Autodesk Inventor part; units mm, degrees
ref_plane "YZ Plane" through (0, 0, 0) normal (1, 0, 0) x (0, 1, 0)
ref_plane "XZ Plane" through (0, 0, 0) normal (0, 1, 0) x (-1, 0, 0)
ref_plane "XY Plane" through (0, 0, 0) normal (0, 0, 1) x (1, 0, 0)
ref_plane "Work Plane1" through (44.003, -30.6729, -33.7942) normal (0, 0, 1) x (1, 0, 0)
sketch "Sketch1" plane through (44.003, -30.6729, -33.7942) normal (0, 0, 1) x (1, 0, 0)
  line L0 (145, 55) -> (160, 55)
  arc A0 (145, 55) -> (135, 45) centre (145, 45) ccw
  line L1 (135, 30) -> (135, 45)
  arc A1 (135, 30) -> (145, 20) centre (145, 30) ccw
  line L2 (160, 20) -> (145, 20)
  arc A2 (160, 20) -> (170, 30) centre (160, 30) ccw
  line L3 (170, 45) -> (170, 30)
  arc A3 (170, 45) -> (160, 55) centre (160, 45) ccw
  point P0 (-44.003, 30.6729)
surface extrude "ExtrusionSrf1" sketch "Sketch1" along normal blind 20 shown yes curves A3 L0 A0 L1 A1 L2 A2 L3
thicken "Thicken1" operation new thickness 3 both sides no extend neighbours no toward (-0.7330519, 0.6801727, 0) faces at (211.3335, -7.4746, -20.4609) (214.003, 4.3271, -27.1276) (210.8047, 21.6576, -20.4609) (199.003, 24.3271, -27.1276) (181.6724, 21.1289, -20.4609) (179.003, 9.3271, -27.1276) (188.2557, -10.6449, -20.4609) (194.003, -10.6729, -27.1276)
properties part number "CE-8.2.2-01-004"
CAD build for the part. Positions are in the model's coordinates, mm. A direction names the side the tool comes from. Coordinates: 2 decimals unless noted, no trailing zeros. Order: outer loops, then holes, each group sorted by start corner. A loop starts at its lowest first (then second) coordinate and runs counter-clockwise, first axis right, second up.
(1) Drill centre lines: L1, parallel to Y at x = 199, z = -21; L2, parallel to X at y = 6.5, z = -15.25; L3, parallel to X at y = -4, z = -24.25. Where is each one in solid material? Low to high.
Solution:
L1: y = -10.67 to -7.67, 21.33 to 24.33
L2: x = 179 to 182, 211 to 214
L3: x = 179.57 to 182.84, 210.16 to 213.43
(2) Saw through at A-A, the plane x = 200. Write the cut outline in (y, z), and give its area (3 significant figures).
Solution:
outline: (-10.67, -33.79) - (-7.67, -33.79) - (-7.67, -13.79) - (-10.67, -13.79) - close; (21.33, -33.79) - (24.33, -33.79) - (24.33, -13.79) - (21.33, -13.79) - close
area: 120 mm2
(3) Mould opens along X. For faces 1 (the face through (214.003, 7, -24)), 2 (the face through (179.003, 7, -24)), 3 (the face through (209.007, -5.568, -23.934)) say: released by +X, released by -X, zero draft, split by the parting line, or undercut.
Solution:
face 1: released by +X
face 2: released by -X
face 3: undercut
(4) Saw through at C-C, the plane z = -25.5. Write the cut outline in (x, y), and give its area (3 significant figures).
Solution:
outline: (179, -0.67) arc R10 ccw to (189, -10.67) - (204, -10.67) arc R10 ccw to (214, -0.67) - (214, 14.33) arc R10 ccw to (204, 24.33) - (189, 24.33) arc R10 ccw to (179, 14.33) - close; hole (182, -0.67) arc R7 ccw to (189, -7.67) - (204, -7.67) arc R7 ccw to (211, -0.67) - (211, 14.33) arc R7 ccw to (204, 21.33) - (189, 21.33) arc R7 ccw to (182, 14.33) - close
area: 340 mm2
(5) Which spindle directions (+Z, -Z, +X, -X, +Y, -Y) get a long thin tool onto all of the face, cutting with end or side? Do faces 4 (the face through (182.01, -7.82, -23.93)), 5 (the face through (183.999, 19.222, -23.934)). Say none if no direction does.
Solution:
face 4: +Z, -Z, -X, -Y
face 5: +Z, -Z
(6) Saw through at B-B, the plane y = 11. Write the cut outline in (x, z).
Solution:
outline: (179, -33.79) - (182, -33.79) - (182, -13.79) - (179, -13.79) - close; (211, -33.79) - (214, -33.79) - (214, -13.79) - (211, -13.79) - close
(7) Pin check, flat tip, straight feed: pin 1 Ø3 at (y, z) = (17, -26.5) entering from -X. Stop position of the tip, or through.
Solution:
pin 1: stops at x = 179.07
